Here's how the part is built. I have some questions about the finished solid (model axes, mm). A direction names the side the tool comes from. Coordinates: 2 decimals unless noted, no trailing zeros. Write each loop counter-clockwise with the first axis right and the second up, starting at its lowest first coordinate (ties: lowest second). Pieces come first, ordered by that corner, then holes. Notation, with made-up numbers: (66.5, 45) - (71.5, 45) arc R19 ccw to (71.5, 70) - close; hole circle Ø4 at (57, -0.75). An arc over 180 degrees is marked (long way). Answer in a Markdown table with one row per item. Add a question column.
Item 1: Imagine slicing it at B-B (z = 61). Please give me the cut outline in (x, y).
Item 2: We'd pull the mould along Y, two halves only. Please class faces 1 (the face through (5.294, 1.667, 32.045)), 2 (the face through (0, 0, 0)), 3 (the face through (3.75, 0.45, 59.57)): +Y half, -Y half, draft (parallel to the pull), parting line (faces both ways), or undercut.
Item 3: Which directions (+Z, -Z, +X, -X, +Y, -Y) give clear straight access to the entire face, cutting with the end or side of a thin tool? Please do faces 4 (the face through (-2, 0, 59)), 5 (the face through (-3, 0, 65)).
Item 4: I'm going to push flat-ended pins straight in: pin 1 (1 mm diameter, centred on x = 1.5, z = 9, fed in from -Y); pin 2 (2 mm diameter, centred on x = -0.5, y = 2.5, fed in from +Z); pin 3 (4 mm diameter, centred on y = 2.5, z = 37.5, fed in from +X). Where does each tip first touch, or does it pass through?
Item 5: If I drill on probe 1 along Z at (x, y) = (-3.8, 0); probe 2 along X at (y, z) = (0.25, 56); probe 3 along Z at (x, y) = (-1, -0.5), over which ranges is the centre line in solid material (lowest first)? Write a range as from..to.
Item 6: Imagine slicing it at D-D (z = 31). Please give me the cut outline in (x, y).
Item 7: Imagine slicing it at C-C (x = 0). Please give me the cut outline in (y, z), plus the area to 3 significant figures.
Item 8: Imagine slicing it at A-A (y = 0). Please give me the cut outline in (x, z).
from build123d import *

# Parameters (mm, degrees)
ESQUISSE1_R                  = 5.55
BOSS_EXTRU_1_DEPTH           = 65
ENL_V_MAT_EXTRU_1_DEPTH      = 12
ESQUISSE3_R                  = 1.5
ENL_V_MAT_EXTRU_2_DEPTH      = 6.55
ENL_V_MAT_EXTRU_2_DEPTH_BACK = 6.55


with BuildPart() as part:
    # Esquisse1 → Boss.-Extru.1 (new body)
    with BuildSketch(Plane.XY):
        Circle(ESQUISSE1_R)
    extrude(amount=BOSS_EXTRU_1_DEPTH)

    # Esquisse2 → Enlèv. mat.-Extru.1 (cut)
    with BuildSketch(Plane.XY.offset(65)):
        with BuildLine():
            Line((-2, 5.177113095), (-2, -5.177113095))
            ThreePointArc((-2, -5.177113095), (0, -5.55), (2, -5.177113095))
            Line((2, -5.177113095), (2, 5.177113095))
            ThreePointArc((2, 5.177113095), (0, 5.55), (-2, 5.177113095))
        make_face()
    extrude(amount=-ENL_V_MAT_EXTRU_1_DEPTH, mode=Mode.SUBTRACT)

    # Esquisse3 → Enlèv. mat.-Extru.2 (cut, two sides)
    with BuildSketch(Plane(origin=(0, 0, 0), x_dir=(0, 0, -1), z_dir=(1, 0, 0))) as enl_v_mat_extru_2_sk:
        with Locations((-61, 0)):
            Circle(ESQUISSE3_R)
    extrude(amount=ENL_V_MAT_EXTRU_2_DEPTH, mode=Mode.SUBTRACT)
    extrude(enl_v_mat_extru_2_sk.sketch, amount=-ENL_V_MAT_EXTRU_2_DEPTH_BACK, mode=Mode.SUBTRACT)


solid = part.part
Here are the results:
| question | item | result |
|---|---|---|
| 1 | outline | (-5.34, -1.5) arc R5.55 ccw to (-2, -5.18) - (-2, -1.5) - close; (-5.34, 1.5) - (-2, 1.5) - (-2, 5.18) arc R5.55 ccw to start; (2, -5.18) arc R5.55 ccw to (5.34, -1.5) - (2, -1.5) - close; (2, 1.5) - (5.34, 1.5) arc R5.55 ccw to (2, 5.18) - close |
| 2 | face 1 | parting line |
| 2 | face 2 | draft |
| 2 | face 3 | undercut |
| 3 | face 4 | +Z, +Y, -Y |
| 3 | face 5 | +Z, +X, -X, +Y, -Y |
| 4 | pin 1 | stops at y = -5.46 |
| 4 | pin 2 | stops at z = 53 |
| 4 | pin 3 | stops at x = 5.53 |
| 5 | probe 1 | z = 0..59.5, 62.5..65 |
| 5 | probe 2 | x = -5.54..-2, 2..5.54 |
| 5 | probe 3 | z = 0..53 |
| 6 | outline | circle Ø11.1 at (0, 0) |
| 7 | outline | (-5.55, 0) - (5.55, 0) - (5.55, 53) - (-5.55, 53) - close |
| 7 | area | 588 mm2 |
| 8 | outline | (-5.55, 0) - (5.55, 0) - (5.55, 59.5) - (2, 59.5) - (2, 53) - (-2, 53) - (-2, 59.5) - (-5.55, 59.5) - close; (-5.55, 62.5) - (-2, 62.5) - (-2, 65) - (-5.55, 65) - close; (2, 62.5) - (5.55, 62.5) - (5.55, 65) - (2, 65) - close |
